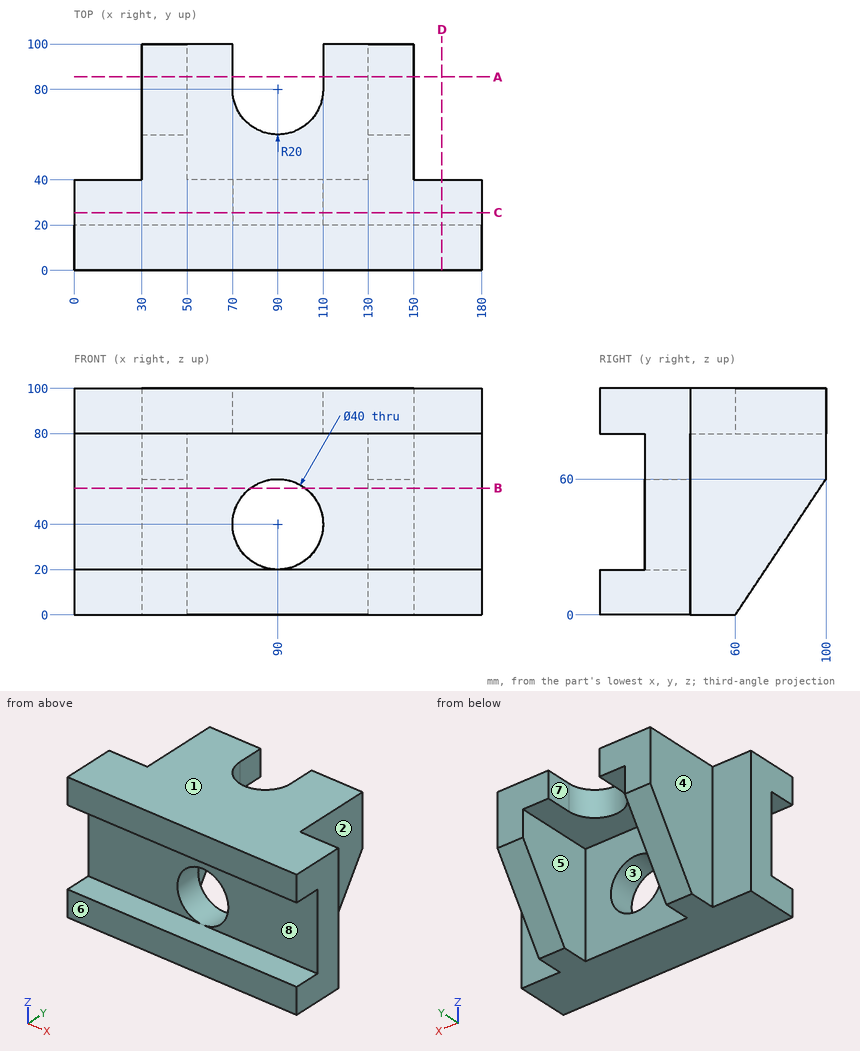
Job drawing, mm, ordinate dimensions from the low corner. One solid piece. A direction names the side the tool comes from. Round coordinates to 2 decimals unless told otherwise and drop trailing zeros. Loops run counter-clockwise (first coordinate to the right, second up) from the corner with the lowest first, then second, coordinate; pieces in that order, holes last. Notation, with made-up numbers: (68.5, 2) -> (79.5, 2) arc R18 ccw to (79.5, 15) -> close; hole circle Ø9 at (49, -40). An arc over 180 degrees is marked (long way). One line per item, written item: value. Start each with the question number.
Q1. Cut at B-B on z = 56. List the corners of the cut face in (x, y).
Q2. Cut at C-C on y = 25.5. List the corners of the cut face in (x, z), plus the area to 3 significant figures.
Q3. 3-axis set-ups, long thin cutter, end or side, ignore diameter. For the marked faces 4, 5, 6, 7 and 8: which of +Z, -Z, +X, -X, +Y, -Y reach the whole face in a straight line?
Q4. Cut at A-A on y = 85.5. List the corners of the cut face in (x, z), plus the area to 3 significant figures.
Q5. Drop flat-ended pins along their axis: pin 1 Ø9 at (x, z) = (168.5, 48) entering from +Y; pin 2 Ø22 at (y, z) = (90, 92) entering from +X; pin 3 Ø10 at (x, y) = (86, 50) entering from -Z. Give the stop position or say it passes through.
Q6. Probe line 1 along Z through (x, y) = (90, 35.5); line 2 along Z through (x, y) = (123, 8); line 3 along X through (y, z) = (69.5, 34). List the from-to ranges inside material, lowest first.
Q7. Two-plate mould, pull along X, no slides. Class the marked faces 1, 2 and 3: released by +X, released by -X, zero draft, split by the parting line, or undercut.
Q8. Cut at D-D on x = 162.5. List the corners of the cut face in (y, z).
Computed:
1. outline: (0, 20) -> (78, 20) -> (78, 40) -> (50, 40) -> (50, 97.33) -> (30, 97.33) -> (30, 40) -> (0, 40) -> close; (102, 20) -> (180, 20) -> (180, 40) -> (150, 40) -> (150, 97.33) -> (130, 97.33) -> (130, 40) -> (102, 40) -> close
2. outline: (0, 0) -> (180, 0) -> (180, 100) -> (0, 100) -> close; hole circle Ø40 at (90, 40)
2. area: 16,700 mm²
3. face 4: +Z, -Z, -X, +Y
3. face 5: -Z, +Y
3. face 6: +Z, -Z, +X, -X, -Y
3. face 7: +Z, -Z, +Y
3. face 8: +X, -X, -Y
4. outline: (30, 38.25) -> (50, 38.25) -> (50, 80) -> (70, 80) -> (70, 100) -> (30, 100) -> close; (110, 80) -> (130, 80) -> (130, 38.25) -> (150, 38.25) -> (150, 100) -> (110, 100) -> close
4. area: 3,270 mm²
5. pin 1: y = 40
5. pin 2: x = 150
5. pin 3: z = 80
6. line 1: 0 to 20, 60 to 100
6. line 2: 0 to 20, 80 to 100
6. line 3: 30 to 50, 130 to 150
7. face 1: zero draft
7. face 2: released by +X
7. face 3: undercut
8. outline: (0, 0) -> (40, 0) -> (40, 100) -> (0, 100) -> (0, 80) -> (20, 80) -> (20, 20) -> (0, 20) -> close
